```python
from build123d import *

# Parameters (mm, degrees)
F0_W     = 30
F0_H     = 10
F1_DEPTH = 2.5
F2_R     = 4
F3_DEPTH = 1
F4_R     = 0.5
F5_DEPTH = 3
F6_R     = 1.25
F7_DEPTH = 5.001
F8_R     = 2


with BuildPart() as f1:
    # F0 (on Top) → F1 (new body, symmetric)
    with BuildSketch(Plane.XY):
        Rectangle(F0_W, F0_H)
    extrude(amount=F1_DEPTH, both=True)

    # F2 (on face) → F3 (cut)
    with BuildSketch(Plane.XY.offset(2.5)):
        with Locations((-10, 0)):
            Circle(F2_R)
    extrude(amount=-F3_DEPTH, mode=Mode.SUBTRACT)

    # F4 (on face) → F5 (cut)
    with BuildSketch(Plane.XY.offset(1.5)):
        with Locations((-11.5, 2)):
            Circle(F4_R)
        with Locations((-8.5, 2)):
            Circle(F4_R)
        with Locations((-10, -2)):
            Circle(F4_R)
    extrude(amount=-F5_DEPTH, mode=Mode.SUBTRACT)

    # F6 (on face) → F7 (cut, through all)
    with BuildSketch(Plane.XY.offset(2.5)):
        with Locations((10, 0)):
            Circle(F6_R)
    extrude(amount=-F7_DEPTH, mode=Mode.SUBTRACT)

    # F8
    f8_edges = [f1.edges().sort_by_distance(p)[0] for p in [
        (-15, -5, 0),
        (-15, 5, 0),
        (15, -5, 0),
        (15, 5, 0),
    ]]
    fillet(f8_edges, radius=F8_R)


solid = f1.part
```
CAD build for the part. Positions are in the model's coordinates, mm. A direction names the side the tool comes from. Give positions to 0.01 mm unless a question says otherwise; leave off trailing zeros. Loops run counter-clockwise (first coordinate to the right, second up) from the corner with the lowest first, then second, coordinate; pieces in that order, holes last. Notation, with made-up numbers: (40.25, 67.5) - (56.25, 67.5) arc R20 ccw to (56.25, 73.5) - close; hole circle Ø9 at (48, 1.5). An arc over 180 degrees is marked (long way). Put each result on its own line as item: value.
Q1. Mould opens along Y. For faces 1 (the face through (15, 0, 0)), 2 (the face through (-13.2, -2.4, 2)), 3 (the face through (0, 5, 0)), 4 (the face through (-8.5, 2, -1.5)) say: pulls with the +Y half, pulls with the -Y half, needs draft (parallel to the pull), parting line crosses it, or undercut.
Filled in:
face 1: needs draft
face 2: undercut
face 3: pulls with the +Y half
face 4: undercut
Q2. Slice it at A-A (x = 10). Give the cut face in (y, z).
Filled in:
outline: (-5, -2.5) - (-1.25, -2.5) - (-1.25, 2.5) - (-5, 2.5) - close; (1.25, -2.5) - (5, -2.5) - (5, 2.5) - (1.25, 2.5) - close
Q3. Probe line 1 along Y through (x, z) = (-8.5, -0.7); line 2 along Y through (x, z) = (-10, 2); line 3 along X through (y, z) = (2.25, -1.15). List the from-to ranges inside material, lowest first.
Filled in:
line 1: y = -5 to 1.5, 2.5 to 5
line 2: y = -5 to -4, 4 to 5
line 3: x = -15 to -11.93, -11.07 to -8.93, -8.07 to 15
Q4. Slice it at D-D (z = 2.1). Give the cut face in (x, y).
Filled in:
outline: (-15, -3) arc R2 ccw to (-13, -5) - (13, -5) arc R2 ccw to (15, -3) - (15, 3) arc R2 ccw to (13, 5) - (-13, 5) arc R2 ccw to (-15, 3) - close; hole circle Ø8 at (-10, 0); hole circle Ø2.5 at (10, 0)
Q5. Flat gauge pins, fed straight in: pin 1 (1.1 mm diameter, centred on x = -10, y = -2, fed in from +Z); pin 2 (0.8 mm diameter, centred on x = -8.5, y = 2, fed in from +Z). Where does each tip first touch, or does it go through?
Filled in:
pin 1: stops at z = 1.5
pin 2: stops at z = -1.5
Q6. Slice it at B-B (z = -0.1). Give the cut face in (x, y).
Filled in:
outline: (-15, -3) arc R2 ccw to (-13, -5) - (13, -5) arc R2 ccw to (15, -3) - (15, 3) arc R2 ccw to (13, 5) - (-13, 5) arc R2 ccw to (-15, 3) - close; hole circle Ø1 at (-11.5, 2); hole circle Ø1 at (-10, -2); hole circle Ø1 at (-8.5, 2); hole circle Ø2.5 at (10, 0)
Q7. Tool access for faces 5 (the face through (-12, 2, 0)), 6 (the face through (-14.43, 4.4, -0.04)): list every direction of +Z, -Z, +X, -X, +Y, -Y with a clear straight run to the whole face (end or side of a thin tool).
Filled in:
face 5: +Z
face 6: +Z, -Z, -X, +Y
Q8. Slice it at C-C (x = -10). Give the cut face in (y, z).
Filled in:
outline: (-5, -2.5) - (5, -2.5) - (5, 2.5) - (4, 2.5) - (4, 1.5) - (-1.5, 1.5) - (-1.5, -1.5) - (-2.5, -1.5) - (-2.5, 1.5) - (-4, 1.5) - (-4, 2.5) - (-5, 2.5) - close
